from build123d import *

# Parameters (mm, degrees)
SKETCH1_R             = 50
SKETCH1_R_2           = 35
BOSS_EXTRUDE1_DEPTH   = 6.35
BOSS_EXTRUDE2_DEPTH   = 6.35
F_6_32_TAPPED_HOLE1_D = 2.7051
FILLET1_R             = 10
M4X0_7_TAPPED_HOLE1_D = 2.8
SKETCH11_W            = 35
SKETCH11_H            = 40
CUT_EXTRUDE1_DEPTH    = 10
FILLET2_R             = 5
M3X0_5_TAPPED_HOLE1_D = 2


with BuildPart() as part:
    # Sketch1 → Boss-Extrude1 (new body)
    with BuildSketch(Plane.XY):
        Circle(SKETCH1_R)
        Circle(SKETCH1_R_2, mode=Mode.SUBTRACT)
    extrude(amount=BOSS_EXTRUDE1_DEPTH)

    # Sketch3 → Boss-Extrude2 (add)
    with BuildSketch(Plane.XY.offset(6.35)):
        with BuildLine():
            ThreePointArc((50, 0), (0, -50), (-50, 0))
            Line((-50, 0), (-50, -117.7))
            Line((-50, -117.7), (50, -117.7))
            Line((50, -117.7), (50, 0))
        make_face()
    extrude(amount=-BOSS_EXTRUDE2_DEPTH)

    # #6-32 Tapped Hole1 (through all)
    with Locations(Plane.XY.offset(6.35)):
        with Locations((-45, 0), (-31.819805153, -31.819805153), (0, -45), (31.819805153, -31.819805153), (45, 0), (31.819805153, 31.819805153), (0, 45), (-31.819805153, 31.819805153)):
            Hole(F_6_32_TAPPED_HOLE1_D / 2)

    # Fillet1
    fillet1_edges = [part.edges().sort_by_distance(p)[0] for p in [
        (-50, -117.7, 3.175),
        (50, -117.7, 3.175),
    ]]
    fillet(fillet1_edges, radius=FILLET1_R)

    # M4x0.7 Tapped Hole1 (through all)
    with Locations(Plane.XY.offset(6.35)):
        with Locations((-30, -107.7), (30, -107.7), (30, -87.7), (-30, -87.7), (30, -67.7), (-30, -67.7)):
            Hole(M4X0_7_TAPPED_HOLE1_D / 2)

    # Sketch11 → Cut-Extrude1 (cut)
    with BuildSketch(Plane(origin=(0, 0, 0), x_dir=(-1, 0, 0), z_dir=(0, 0, -1))):
        with Locations((-0.110004591, -77.7)):
            Rectangle(SKETCH11_W, SKETCH11_H)
    extrude(amount=-CUT_EXTRUDE1_DEPTH, mode=Mode.SUBTRACT)

    # Fillet2
    fillet2_edges = [part.edges().sort_by_distance(p)[0] for p in [
        (-17.389995409, -57.7, 3.175),
        (-17.389995409, -97.7, 3.175),
        (17.610004591, -97.7, 3.175),
        (17.610004591, -57.7, 3.175),
    ]]
    fillet(fillet2_edges, radius=FILLET2_R)

    # M3x0.5 Tapped Hole1 (through all)
    with Locations(Plane(origin=(0, 0, 0), x_dir=(-1, 0, 0), z_dir=(0, 0, -1))):
        with Locations((-22.610004591, -62.7), (-22.610004591, -92.7), (22.389995409, -92.7), (22.389995409, -62.7)):
            Hole(M3X0_5_TAPPED_HOLE1_D / 2)


solid = part.part
Can you work these out from the model? Positions are in its coordinate system, mm. A direction names the side the tool comes from. Give positions to 0.01 mm unless a question says otherwise; leave off trailing zeros. Loops run counter-clockwise (first coordinate to the right, second up) from the corner with the lowest first, then second, coordinate; pieces in that order, holes last. Notation, with made-up numbers: M 9.5,71 L 42.5,71 A32 ccw 42.5,105 Z; hole C 42.25,71.5 d2. An arc over 180 degrees is marked long. One line per item, written item: value. Start each with the question number.
1) Thinking about a two-plate mould opening in X: for faces 3 (the face through (0, -57.7, 3)), 4 (the face through (-1, -51, 0)), 5 (the face through (-47.15, -114.69, 3.13)), which applies, +X half, -X half, draft (parallel to the pull), parting line (faces both ways), or undercut?
2) If we section it at C-C, the plane x = 14.5: Write out the boundary of the cut face in (y, z), and give its area (3 significant figures).
3) If we section it at D-D, the plane z = 1: Give the number of separate pieces and of enclosed holes in the cut face, and give its area (3 significant figures).
4) If we section it at A-A, the plane x = -19.5: Write out the boundary of the cut face in (y, z), and give its area (3 significant figures).
5) I'm going to push flat-ended pins straight in: pin 1 (3 mm diameter, centred on x = 30, y = -87.7, fed in from +Z); pin 2 (1 mm diameter, centred on y = 10, z = 1.5, fed in from +X); pin 3 (2 mm diameter, centred on x = -0.5, z = 2.5, fed in from +Y). Where does each tip first touch, or does it pass through?
6) If I drill on line 1 (X direction, y = -87.7, z = 4); line 2 (X direction, y = -92.7, z = 5.25); line 3 (Y direction, x = 0, z = 1.5), over which ranges is the centre line in solid material (lowest first)? Write a range as [from, to].
7) On a 3-axis mill with a long thin cutter (end or side, diameter ignored), from which of +Z, -Z, +X, -X, +Y, -Y can I reach the whole of each face in a straight line? I mean faces 1 (the face through (-50, -53, 3)), 2 (the face through (-15.89, -59.13, 3.22)). Say none if no direction works.
8) If we section it at B-B, the plane y = 25: Write out the boundary of the cut face in (x, z).
Completed:
1. face 3: undercut
1. face 4: draft
1. face 5: -X half
2. outline: M -117.7,0 L -97.33,0 L -97.33,6.35 L -117.7,6.35 Z; M -58.07,0 L -31.86,0 L -31.86,6.35 L -58.07,6.35 Z; M 31.86,0 L 47.85,0 L 47.85,6.35 L 31.86,6.35 Z
2. area: 397 mm^2
3. separate pieces: 1
3. enclosed holes: 20
3. area: 10,300 mm^2
4. outline: M -117.7,0 L -29.06,0 L -29.06,6.35 L -117.7,6.35 Z; M 29.06,0 L 46.04,0 L 46.04,6.35 L 29.06,6.35 Z
4. area: 671 mm^2
5. pin 1: stops at z = 6.35
5. pin 2: stops at x = 49.09
5. pin 3: stops at y = 50
6. line 1: x = [-50, -31.4], [-28.6, -17.39], [17.61, 28.6], [31.4, 50]
6. line 2: x = [-50, -23.39], [-21.39, -17.39], [17.61, 21.61], [23.61, 50]
6. line 3: y = [-117.7, -97.7], [-57.7, -46.35], [-43.65, -35], [35, 43.65], [46.35, 50]
7. face 1: +Z, -Z, -X, +Y, -Y
7. face 2: +Z, -Z
8. outline: M -43.3,0 L -24.49,0 L -24.49,6.35 L -43.3,6.35 Z; M 24.49,0 L 43.3,0 L 43.3,6.35 L 24.49,6.35 Z
